Work out the finished part from the listing and answer in its coordinate system (mm). A direction names the side the tool comes from. Give positions to 0.01 mm unless a question says otherwise; leave off trailing zeros. Loops run counter-clockwise (first coordinate to the right, second up) from the corner with the lowest first, then second, coordinate; pieces in that order, holes last. Notation, with made-up numbers: (24.25, 30.5) - (43.25, 30.5) arc R14 ccw to (43.25, 57.5) - close; hole circle Ø4 at (-31.75, -28.75). An arc over 180 degrees is marked (long way). Use CSV: the item, a comma, the result in double quotes.
from build123d import *

# Parameters (mm, degrees)
SKETCH1_W           = 25
SKETCH1_H           = 15
SKETCH1_R           = 1
BOSS_EXTRUDE1_DEPTH = 5
SKETCH2_R           = 1.875
CUT_EXTRUDE1_DEPTH  = 3.3
CUT_EXTRUDE2_DEPTH  = 6
SKETCH4_W           = 25
SKETCH4_H           = 5
BOSS_EXTRUDE2_DEPTH = 31.8
SKETCH5_R           = 1
CUT_EXTRUDE3_DEPTH  = 6
SKETCH8_R           = 1.875
CUT_EXTRUDE4_DEPTH  = 1.25
CIRPATTERN1_COUNT   = 4
SKETCH9_R           = 4.05
CUT_EXTRUDE5_DEPTH  = 6
FILLET1_R           = 2
FILLET2_R           = 2


with BuildPart() as part:
    # Sketch1 → Boss-Extrude1 (new body)
    with BuildSketch(Plane.XY):
        with Locations((12.5, 7.5)):
            Rectangle(SKETCH1_W, SKETCH1_H)
        with Locations((4.5, 3.5)):
            Circle(SKETCH1_R, mode=Mode.SUBTRACT)
        with Locations((20.5, 3.5)):
            Circle(SKETCH1_R, mode=Mode.SUBTRACT)
    extrude(amount=BOSS_EXTRUDE1_DEPTH)

    # Sketch2 → Cut-Extrude1 (cut)
    with BuildSketch(Plane(origin=(0, 0, 0), x_dir=(-1, 0, 0), z_dir=(0, 0, -1))):
        with Locations((-20.5, 3.5)):
            Circle(SKETCH2_R)
        with Locations((-4.5, 3.5)):
            Circle(SKETCH2_R)
    extrude(amount=-CUT_EXTRUDE1_DEPTH, mode=Mode.SUBTRACT)

    # Sketch3 → Cut-Extrude2 (cut, through all)
    with BuildSketch(Plane(origin=(0, 0, 0), x_dir=(-1, 0, 0), z_dir=(0, 0, -1))):
        Polygon((0, 0), (-3.5, 0), (0, 3.5), align=None)
        Polygon((-21.5, 0), (-25, 0), (-25, 3.5), align=None)
    extrude(amount=-CUT_EXTRUDE2_DEPTH, mode=Mode.SUBTRACT)


with BuildPart() as body_2:
    # Mirror5: mirrored copy
    add(part.part.mirror(Plane.XY.offset(20.9)))


with BuildPart() as part_1:
    add(part.part)

    add(body_2.part)  # Boss-Extrude2 merges body 2
    # Sketch4 → Boss-Extrude2 (add)
    with BuildSketch(Plane(origin=(0, 0, 36.8), x_dir=(-1, 0, 0), z_dir=(0, 0, -1))):
        with Locations((-12.5, 12.5)):
            Rectangle(SKETCH4_W, SKETCH4_H)
    extrude(amount=BOSS_EXTRUDE2_DEPTH)

    # Sketch5 → Cut-Extrude3 (cut, through all)
    with BuildSketch(Plane.XZ.offset(-10)):
        with Locations((20.5, 20.9)):
            Circle(SKETCH5_R)
    cut_extrude3 = extrude(amount=-CUT_EXTRUDE3_DEPTH, mode=Mode.SUBTRACT)

    # Sketch8 → Cut-Extrude4 (cut)
    with BuildSketch(Plane.XZ.offset(-10)):
        with Locations((20.5, 20.9)):
            Circle(SKETCH8_R)
    cut_extrude4 = extrude(amount=-CUT_EXTRUDE4_DEPTH, mode=Mode.SUBTRACT)

    # CirPattern1: Cut-Extrude3, Cut-Extrude4 ×4 about axis
    cirpattern1_axis = Axis((12.5, 0, 20.9), (0, 1, 0))
    for i in range(1, CIRPATTERN1_COUNT):
        add(cut_extrude3.rotate(cirpattern1_axis, i * 360 / CIRPATTERN1_COUNT), mode=Mode.SUBTRACT)
        add(cut_extrude4.rotate(cirpattern1_axis, i * 360 / CIRPATTERN1_COUNT), mode=Mode.SUBTRACT)

    # Sketch9 → Cut-Extrude5 (cut, through all)
    with BuildSketch(Plane.XZ.offset(-10)):
        with Locations((12.5, 20.9)):
            Circle(SKETCH9_R)
    extrude(amount=-CUT_EXTRUDE5_DEPTH, mode=Mode.SUBTRACT)

    # Fillet1
    fillet1_edges = [part_1.edges().sort_by_distance(p)[0] for p in [
        (12.5, 10, 36.8),
    ]]
    fillet(fillet1_edges, radius=FILLET1_R)

    # Fillet2
    fillet2_edges = [part_1.edges().sort_by_distance(p)[0] for p in [
        (12.5, 10, 5),
    ]]
    fillet(fillet2_edges, radius=FILLET2_R)


solid = part_1.part
Item 1: For faces 1 (the flat face through (12, 8, 41.8)), 2 (the flat face through (5, 2, 3.3)), 3 (the flat face through (5, 2, 38.5)), 4 (the flat face through (12, 4, 5)), 5 (the flat face through (4, 11.25, 22)), determine the directions among +Z, -Z, +X, -X, +Y, -Y from which every point of the face is accessible in a straight line to the end or side of a thin tool.
Determined:
face 1,"+Z, +X, -X, +Y, -Y"
face 2,"-Z"
face 3,"+Z"
face 4,"+X, -X, -Y"
face 5,"-Y"
Item 2: The mould has two halves that part along Y. Classify faces 6 (the flat face through (15.5, 10, 24.2)), 7 (the cylindrical face through (12.117, 13.099, 11.976)), 8 (the cylindrical face through (22.373, 3.582, 1.627)): pulls with the +Y half, pulls with the -Y half, needs draft (parallel to the pull), parting line crosses it, or undercut.
Determined:
face 6,"pulls with the -Y half"
face 7,"needs draft"
face 8,"undercut"
Item 3: Given P1, Ø1.9, axis at x = 20, y = 3.5, coming from the -Z side; P2, Ø2.5, axis at x = 4.5, y = 3.5, coming from the +Z side; P3, Ø3, axis at x = 4.5, z = 21, coming from the -Y side, each flat-ended and moving along its own axis, determine where each tip first touches the part or whether it passes through.
Determined:
P1,"stops at z = 3.3"
P2,"stops at z = 38.5"
P3,"stops at y = 11.25"
Item 4: A cutting plane is placed at B-B on y = 12.75. Determine the outline of the cut face in (x, z), and give its area (3 significant figures).
Determined:
outline,"(0, 0) - (25, 0) - (25, 41.8) - (0, 41.8) - close; hole circle Ø2 at (4.5, 20.9); hole circle Ø8.1 at (12.5, 20.9); hole circle Ø2 at (12.5, 12.9); hole circle Ø2 at (12.5, 28.9); hole circle Ø2 at (20.5, 20.9)"
area,"981 mm²"
Item 5: A cutting plane is placed at A-A on x = 12.5. State how many separate pieces and enclosed holes the cut face has, and give its area (3 significant figures).
Determined:
separate pieces,"4"
enclosed holes,"0"
area,"246 mm²"
Item 6: A cutting plane is placed at C-C on z = 20.9. Determine the outline of the cut face in (x, y) (3 decimals).
Determined:
outline,"(0, 10) - (2.625, 10) - (2.625, 11.25) - (3.5, 11.25) - (3.5, 15) - (0, 15) - close; (5.5, 11.25) - (6.375, 11.25) - (6.375, 10) - (8.45, 10) - (8.45, 15) - (5.5, 15) - close; (16.55, 10) - (18.625, 10) - (18.625, 11.25) - (19.5, 11.25) - (19.5, 15) - (16.55, 15) - close; (21.5, 11.25) - (22.375, 11.25) - (22.375, 10) - (25, 10) - (25, 15) - (21.5, 15) - close"
Item 7: A cutting plane is placed at D-D on y = 6.5. Determine the outline of the cut face in (x, z), and give its area (3 significant figures).
Determined:
outline,"(0, 0) - (25, 0) - (25, 5) - (0, 5) - close; (0, 36.8) - (25, 36.8) - (25, 41.8) - (0, 41.8) - close"
area,"250 mm²"
Item 8: Find the intervals of material crossed by line 1 (Z direction, x = 19, y = 5); line 2 (X direction, y = 3.5, z = 38.1); line 3 (Y direction, x = 20.5, z = 38), in increasing order.
Determined:
line 1,"z = 0 to 5, 36.8 to 41.8"
line 2,"x = 0 to 3.5, 5.5 to 19.5, 21.5 to 25"
line 3,"y = 0 to 2.5, 4.5 to 15"
